Autodesk Inventor part; units mm, degrees
ref_plane "Work Plane1" through (0, 0, 30.1) normal (0, 0, -1) x (-1, 0, 0)
ref_plane "YZ Plane" through (0, 0, 0) normal (1, 0, 0) x (0, 1, 0)
ref_plane "XZ Plane" through (0, 0, 0) normal (0, 1, 0) x (-1, 0, 0)
sketch "Sketch1" plane through (0, 0, 0) normal (0, 0, 1) x (1, 0, 0)
  line L0 (0, 0) -> (-19.215, 0)
  line L1 (-19.215, 0) -> (-19.215, 7.2)
  line L2 (-16.215, 10.2) -> (-15.215, 10.2)
  line L3 (0, 10.2) -> (0, 2)
  arc A0 (-16.215, 10.2) -> (-19.215, 7.2) centre (-16.215, 7.2) ccw
  line L4 (-15.215, 10.2) -> (-15.215, 2)
  line L5 (-15.215, 2) -> (0, 2)
  line L6 (-15.215, 10.2) -> (0, 10.2)
  line L7 (0, 2) -> (0, 0)
  line L8 (-15.215, 10.2) -> (-15.215, 13.2)
  line L9 (-22.215, 0) -> (-22.215, 9.2)
  line L10 (-18.215, 13.2) -> (-15.215, 13.2)
  arc A1 (-18.215, 13.2) -> (-22.215, 9.2) centre (-18.215, 9.2) ccw
  line L11 (-22.215, 0) -> (-19.215, 0)
  line L12 (0, 0) -> (2, 0)
  line L13 (2, 0) -> (2, 2)
  line L14 (2, 2) -> (0, 2)
  line L15 (0, 2) -> (0, 0)
  dimension "d0" = 3
  dimension "d1" = 19.215
  dimension "d2" = 10.2
  dimension "d3" = 4
  dimension "d4" = 2
  dimension "d5" = 3
  dimension "d6" = 3
  dimension "d7" = 4
  dimension "d10" = 2
  dimension "d11" = 2
extrude "Extrusion1" add sketch "Sketch1" along normal blind 60.2 contours L7 L14 L13 L12 | L11 L9 A1 L10 L8 L2 A0 L1
sketch "Sketch2" plane through (0, 0, 60.2) normal (0, 0, 1) x (1, 0, 0)
  line L0 (-15.215, 10.2) -> (-15.215, 13.2)
  line L1 (-15.215, 13.2) -> (-18.215, 13.2)
  arc A0 (-18.215, 13.2) -> (-22.215, 9.2) centre (-18.215, 9.2) ccw
  line L2 (-22.215, 9.2) -> (-22.215, 0)
  line L3 (-22.215, 0) -> (-19.215, 0)
  line L4 (-19.215, 0) -> (-19.215, 7.2)
  arc A1 (-16.215, 10.2) -> (-19.215, 7.2) centre (-16.215, 7.2) ccw
  line L5 (-16.215, 10.2) -> (-15.215, 10.2)
  line L6 (0, 2) -> (0, 0)
  line L7 (0, 0) -> (2, 0)
  line L8 (2, 0) -> (2, 2)
  line L9 (2, 2) -> (0, 2)
  line L10 (0, 2) -> (-19.215, 2)
  line L11 (-19.215, 0) -> (0, 0)
  line L12 (-15.215, 10.2) -> (0, 2)
extrude "Extrusion2" add sketch "Sketch2" along normal blind 3
sketch "Sketch3" plane through (0, 0, 0) normal (0, 0, -1) x (-1, 0, 0)
  line L0 (0, 2) -> (0, 0)
  line L1 (-2, 2) -> (0, 2)
  line L2 (-2, 0) -> (-2, 2)
  line L3 (0, 0) -> (-2, 0)
  line L4 (19.215, 0) -> (19.215, 7.2)
  line L5 (0, 2) -> (0, 0)
  line L6 (19.215, 0) -> (0, 0)
  line L7 (15.215, 10.2) -> (15.215, 13.2)
  line L8 (16.215, 10.2) -> (15.215, 10.2)
  arc A0 (19.215, 7.2) -> (16.215, 10.2) centre (16.215, 7.2) ccw
  line L9 (19.215, 0) -> (19.215, 7.2)
  line L10 (22.215, 0) -> (19.215, 0)
  line L11 (22.215, 9.2) -> (22.215, 0)
  arc A1 (22.215, 9.2) -> (18.215, 13.2) centre (18.215, 9.2) ccw
  line L12 (15.215, 13.2) -> (18.215, 13.2)
  line L13 (16.215, 10.2) -> (15.215, 10.2)
  line L14 (0, 2) -> (15.215, 10.2)
  arc A2 (19.215, 7.2) -> (16.215, 10.2) centre (16.215, 7.2) ccw
extrude "Extrusion3" add sketch "Sketch3" along normal blind 3
sketch "Sketch4" plane through (-22.215, 0, 63.2) normal (0, -1, 0) x (1, 0, 0)
  circle A0 centre (12.1075, 4) radius 2
  line L0 (3, -63.2) -> (3, -3)
  line L1 (3, -3) -> (22.215, -3)
  line L2 (22.215, -63.2) -> (22.215, -3)
  line L3 (22.215, -63.2) -> (3, -63.2)
  line L4 (0, -66.2) -> (0, 0)
  line L5 (24.215, -66.2) -> (0, -66.2)
  line L6 (24.215, -66.2) -> (24.215, 0)
  line L7 (0, 0) -> (24.215, 0)
  line L8 (12.1075, 0) -> (12.1075, 4) construction
  arc A1 (12.1075, 0) -> (16.1075, 4) centre (12.1075, 4) ccw construction
  line L9 (8.1075, 4) -> (8.1075, 0)
  line L10 (16.1075, 4) -> (16.1075, 0)
  arc A2 (8.1075, 4) -> (12.1075, 0) centre (12.1075, 4) ccw construction
  arc A3 (16.1075, 4) -> (8.1075, 4) centre (12.1075, 4) ccw
  dimension "d16" = 4
  dimension "d17" = 4
extrude "Extrusion4" add sketch "Sketch4" against normal up to surface (2 mm away) contours L9 A3 L10 L7
ref_plane "Work Plane1" through (0, 0, 30.1) normal (0, 0, -1) x (-1, 0, 0)
mirror "Mirror1" about plane through (0, 0, 30.1) normal (0, 0, -1) of "Extrusion4"
fillet "Fillet1" radius 3 4 edges at (-14.1075, 1, -3) (-6.1075, 1, -3) (-6.1075, 1, 63.2) (-14.1075, 1, 63.2)
properties part number "Clamp_Holder"
Design review of the part built by this model. Coordinates are the model's own, in mm. A direction names the side the tool comes from. Round coordinates to 2 decimals unless told otherwise and drop trailing zeros. Write each loop counter-clockwise with the first axis right and the second up, starting at its lowest first coordinate (ties: lowest second). Pieces come first, ordered by that corner, then holes. Notation, with made-up numbers: (49, 39.5) - (95, 39.5) arc R5 cw to (95, 46.5) - close; hole circle Ø5 at (-32.5, 76.25). An arc over 180 degrees is marked (long way). Use a Markdown table: item, result. Add a question column.
1. Clearance check with flat-ended pins moving along their axes: pin 1 (0.6 mm diameter, centred on x = 1.5, z = 36, fed in from +Y); pin 2 (5 mm diameter, centred on x = -5, y = 5, fed in from +Z); pin 3 (3 mm diameter, centred on x = -19.5, z = 48.5, fed in from +Y); pin 4 (1.1 mm diameter, centred on x = -15.5, z = 36.5, fed in from -Y). State where each tip first meets the part, or that it passes through.
2. Wall thickness on probe 1 along X at (y, z) = (1.1, -7); probe 2 along Z at (x, y) = (-3.5, 3.75); probe 3 along Y at (x, z) = (1, 52): over which ranges is each line inside the solid? List them lowest first.
3. Mouldability with a two-part tool opening along Z and no side actions: class faces 3 (the face through (0, 1, 30)), 4 (the face through (1, 2, 30)), 5 (the face through (-10, 1, 71.2)) as +Z half, -Z half, draft (parallel to the pull), parting line (faces both ways), or undercut.
4. We need section B-B (x = -7). State the section outline as (y, z) points, then the cut area to 3 significant figures.
5. For faces 1 (the face through (-12, 4, 0)), 2 (the face through (-14.963, 1.014, 64.102)), list the 3-axis set-ups (+Z, -Z, +X, -X, +Y, -Y) from which the entire face can be reached by the end or side of a thin tool; tool diameter is ignored.
6. We need section C-C (z = 61). State the section outline as (x, y) points (3 decimals).
7. We need section A-A (z = 12.5). State the section outline as (x, y) points (3 decimals).
8. We need section D-D (y = 2.75). State the section outline as (x, z) points (3 decimals).
Output:
| question | item | result |
|---|---|---|
| 1 | pin 1 | stops at y = 2 |
| 1 | pin 2 | stops at z = 63.2 |
| 1 | pin 3 | stops at y = 13.2 |
| 1 | pin 4 | stops at y = 10.2 |
| 2 | probe 1 | x = -14.11 to -12.11, -8.11 to -6.11 |
| 2 | probe 2 | z = -3 to 0, 60.2 to 63.2 |
| 2 | probe 3 | y = 0 to 2 |
| 3 | face 3 | undercut |
| 3 | face 4 | draft |
| 3 | face 5 | +Z half |
| 4 | outline | (0, -9.52) - (2, -9.52) - (2, -3) - (5.77, -3) - (5.77, 0) - (0, 0) - close; (0, 60.2) - (5.77, 60.2) - (5.77, 63.2) - (2, 63.2) - (2, 69.72) - (0, 69.72) - close |
| 4 | area | 60.7 mm2 |
| 5 | face 1 | -Y |
| 5 | face 2 | +Z, -X, +Y, -Y |
| 6 | outline | (-22.215, 0) - (2, 0) - (2, 2) - (0, 2) - (-15.215, 10.2) - (-15.215, 13.2) - (-18.215, 13.2) arc R4 ccw to (-22.215, 9.2) - close |
| 7 | outline | (-22.215, 0) - (-19.215, 0) - (-19.215, 7.2) arc R3 cw to (-16.215, 10.2) - (-15.215, 10.2) - (-15.215, 13.2) - (-18.215, 13.2) arc R4 ccw to (-22.215, 9.2) - close; (0, 0) - (2, 0) - (2, 2) - (0, 2) - close |
| 8 | outline | (-22.215, -3) - (-1.392, -3) - (-1.392, 0) - (-19.215, 0) - (-19.215, 60.2) - (-1.392, 60.2) - (-1.392, 63.2) - (-22.215, 63.2) - close |
